```python
from build123d import *

# Parameters (mm, degrees)
SALIENTE_EXTRUIR1_DEPTH = 40
REDONDEO1_R             = 0.5
CROQUIS5_W              = 30
CROQUIS5_H              = 220
CORTAR_EXTRUIR2_DEPTH   = 5
CORTAR_EXTRUIR3_REACH   = 211.557
CROQUIS6_R              = 4
CROQUIS6_R_2            = 2.9
REDONDEO2_R             = 0.5


with BuildPart() as part:
    # Croquis2 → Saliente-Extruir1 (new body)
    with BuildSketch(Plane(origin=(0, 0, 0), x_dir=(0, 0, -1), z_dir=(1, 0, 0))):
        Polygon((-24.94884824, -14.646248332), (-12.94884824, -14.646248332), (-12.94884824, -5.646248332), (-12.94884824, 205.353751668), (-24.94884824, 205.353751668), align=None)
    extrude(amount=SALIENTE_EXTRUIR1_DEPTH)

    # Redondeo1
    redondeo1_edges = [part.edges().sort_by_distance(p)[0] for p in [
        (40, 95.353751668, 12.94884824),
        (40, 205.353751668, 18.94884824),
        (40, 95.353751668, 24.94884824),
        (0, 205.353751668, 18.94884824),
        (0, 95.353751668, 12.94884824),
        (0, -14.646248332, 18.94884824),
        (0, 95.353751668, 24.94884824),
        (40, -14.646248332, 18.94884824),
        (20, 205.353751668, 24.94884824),
        (20, 205.353751668, 12.94884824),
        (20, -14.646248332, 12.94884824),
        (20, -14.646248332, 24.94884824),
    ]]
    fillet(redondeo1_edges, radius=REDONDEO1_R)

    # Croquis5 → Cortar-Extruir2 (cut)
    with BuildSketch(Plane.XY.offset(12.94884824)):
        with Locations((20, 95.353751668)):
            Rectangle(CROQUIS5_W, CROQUIS5_H)
    extrude(amount=CORTAR_EXTRUIR2_DEPTH, mode=Mode.SUBTRACT)

    # Croquis6 → Cortar-Extruir3 (cut, up to next)
    with BuildSketch(Plane.XY.offset(24.94884824), mode=Mode.PRIVATE) as cortar_extruir3_sk1:
        with Locations((20, -4.146248332)):
            Circle(CROQUIS6_R)
    cortar_extruir3_tool1 = extrude(cortar_extruir3_sk1.sketch, amount=-CORTAR_EXTRUIR3_REACH, mode=Mode.PRIVATE) & part.part
    # Croquis6 → Cortar-Extruir3 (cut, up to next)
    with BuildSketch(Plane.XY.offset(24.94884824), mode=Mode.PRIVATE) as cortar_extruir3_sk2:
        with Locations((20, 194.853751668)):
            Circle(CROQUIS6_R_2)
    cortar_extruir3_tool2 = extrude(cortar_extruir3_sk2.sketch, amount=-CORTAR_EXTRUIR3_REACH, mode=Mode.PRIVATE) & part.part
    # Croquis6 → Cortar-Extruir3 (cut, up to next)
    with BuildSketch(Plane.XY.offset(24.94884824), mode=Mode.PRIVATE) as cortar_extruir3_sk3:
        with Locations((20, 10.853751668)):
            Circle(CROQUIS6_R)
    cortar_extruir3_tool3 = extrude(cortar_extruir3_sk3.sketch, amount=-CORTAR_EXTRUIR3_REACH, mode=Mode.PRIVATE) & part.part
    # Croquis6 → Cortar-Extruir3 (cut, up to next)
    with BuildSketch(Plane.XY.offset(24.94884824), mode=Mode.PRIVATE) as cortar_extruir3_sk4:
        with Locations((20, 25.853751668)):
            Circle(CROQUIS6_R)
    cortar_extruir3_tool4 = extrude(cortar_extruir3_sk4.sketch, amount=-CORTAR_EXTRUIR3_REACH, mode=Mode.PRIVATE) & part.part
    # Croquis6 → Cortar-Extruir3 (cut, up to next)
    with BuildSketch(Plane.XY.offset(24.94884824), mode=Mode.PRIVATE) as cortar_extruir3_sk5:
        with Locations((20, 40.853751668)):
            Circle(CROQUIS6_R)
    cortar_extruir3_tool5 = extrude(cortar_extruir3_sk5.sketch, amount=-CORTAR_EXTRUIR3_REACH, mode=Mode.PRIVATE) & part.part
    # Croquis6 → Cortar-Extruir3 (cut, up to next)
    with BuildSketch(Plane.XY.offset(24.94884824), mode=Mode.PRIVATE) as cortar_extruir3_sk6:
        with Locations((20, 55.853751668)):
            Circle(CROQUIS6_R)
    cortar_extruir3_tool6 = extrude(cortar_extruir3_sk6.sketch, amount=-CORTAR_EXTRUIR3_REACH, mode=Mode.PRIVATE) & part.part
    add(cortar_extruir3_tool1.solids().sort_by_distance((20, -4.146248, 24.948848))[0], mode=Mode.SUBTRACT)
    add(cortar_extruir3_tool2.solids().sort_by_distance((20, 194.853752, 24.948848))[0], mode=Mode.SUBTRACT)
    add(cortar_extruir3_tool3.solids().sort_by_distance((20, 10.853752, 24.948848))[0], mode=Mode.SUBTRACT)
    add(cortar_extruir3_tool4.solids().sort_by_distance((20, 25.853752, 24.948848))[0], mode=Mode.SUBTRACT)
    add(cortar_extruir3_tool5.solids().sort_by_distance((20, 40.853752, 24.948848))[0], mode=Mode.SUBTRACT)
    add(cortar_extruir3_tool6.solids().sort_by_distance((20, 55.853752, 24.948848))[0], mode=Mode.SUBTRACT)

    # Redondeo2
    redondeo2_edges = [part.edges().sort_by_distance(p)[0] for p in [
        (35, 205.207305058, 13.095294849),
        (5, 205.207305058, 13.095294849),
        (35, 205.353751668, 15.69884824),
        (5, 95.353751668, 12.94884824),
        (5, -14.499801723, 13.095294849),
        (5, 205.353751668, 15.69884824),
        (5, -14.646248332, 15.69884824),
        (35, -14.646248332, 15.69884824),
        (35, -14.499801723, 13.095294849),
        (35, 95.353751668, 12.94884824),
        (5, 95.353751668, 17.94884824),
        (20, -14.646248332, 17.94884824),
        (35, 95.353751668, 17.94884824),
        (20, 205.353751668, 17.94884824),
    ]]
    fillet(redondeo2_edges, radius=REDONDEO2_R)


solid = part.part
```
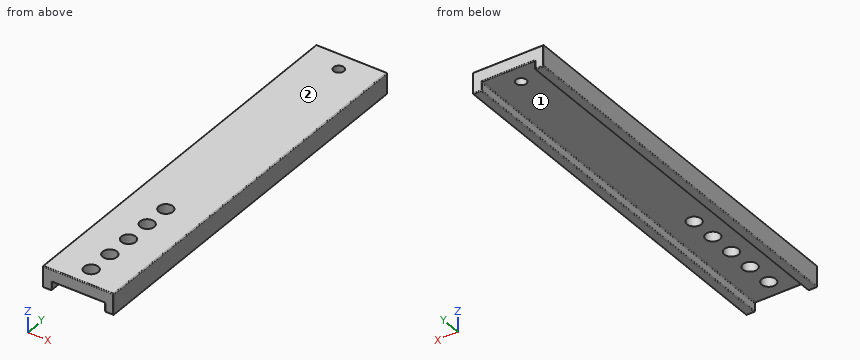
Could you check a few things on this model? Use its own coordinates, in mm. Face numbers are marked on the shaded views. Round coordinates to 2 decimals unless told otherwise and drop trailing zeros. Loops run counter-clockwise (first coordinate to the right, second up) from the corner with the lowest first, then second, coordinate; pieces in that order, holes last.
Q1. For P1, Ø8.5, axis at x = 19, y = 54.5, coming from the -Z side, with a flat end and sliding along its axis, tell me the tip position at first contact or that it passes through.
Q2. I want a section at C-C (x = 30). Write out the boundary of the cut face in (y, z), and give its area (3 significant figures).
Q3. Thinking about a two-plate mould opening in X: for the marked faces 1 and 2, which applies, pulls with the +X half, pulls with the -X half, needs draft (parallel to the pull), parting line crosses it, or undercut?
Q4. I want a section at B-B (y = 43). Write out the boundary of the cut face in (x, z), and give its area (3 significant figures).
Q5. I want a section at A-A (x = 20). Give the number of separate pieces and of enclosed holes in the cut face, and give its area (3 significant figures).
Q6. I want a section at D-D (y = 132). Write out the boundary of the cut face in (x, z).
Q7. Please list where these lines run through material, in increasing order: L1, parallel to X at y = 91.5, z = 14; L2, parallel to Z at x = 18, y = 100; L3, parallel to X at y = 125.5, z = 24.5.
Answer below:
1. P1: stops at z = 17.95
2. outline: (-14.65, 18.45) arc R0.5 ccw to (-14.15, 17.95) - (204.85, 17.95) arc R0.5 ccw to (205.35, 18.45) - (205.35, 24.45) arc R0.5 ccw to (204.85, 24.95) - (-14.15, 24.95) arc R0.5 ccw to (-14.65, 24.45) - close
2. area: 1,540 mm2
3. face 1: undercut
3. face 2: needs draft
4. outline: (0, 13.45) arc R0.5 ccw to (0.5, 12.95) - (4.5, 12.95) arc R0.5 ccw to (5, 13.45) - (5, 17.45) arc R0.5 cw to (5.5, 17.95) - (16.62, 17.95) - (16.62, 24.95) - (0.5, 24.95) arc R0.5 ccw to (0, 24.45) - close; (23.38, 17.95) - (34.5, 17.95) arc R0.5 cw to (35, 17.45) - (35, 13.45) arc R0.5 ccw to (35.5, 12.95) - (39.5, 12.95) arc R0.5 ccw to (40, 13.45) - (40, 24.45) arc R0.5 ccw to (39.5, 24.95) - (23.38, 24.95) - close
4. area: 283 mm2
5. separate pieces: 7
5. enclosed holes: 0
5. area: 1,220 mm2
6. outline: (0, 13.45) arc R0.5 ccw to (0.5, 12.95) - (4.5, 12.95) arc R0.5 ccw to (5, 13.45) - (5, 17.45) arc R0.5 cw to (5.5, 17.95) - (34.5, 17.95) arc R0.5 cw to (35, 17.45) - (35, 13.45) arc R0.5 ccw to (35.5, 12.95) - (39.5, 12.95) arc R0.5 ccw to (40, 13.45) - (40, 24.45) arc R0.5 ccw to (39.5, 24.95) - (0.5, 24.95) arc R0.5 ccw to (0, 24.45) - close
7. L1: x = 0 to 5, 35 to 40
7. L2: z = 17.95 to 24.95
7. L3: x = 0 to 40
